from build123d import *

# Parameters (mm, degrees)
ESBO_O2_R                  = 1.65
RESSALTO_EXTRUS_O1_DEPTH   = 18
CORTE_EXTRUS_O1_DEPTH      = 47.043457733
CORTE_EXTRUS_O1_DEPTH_BACK = 47.043457733
ESBO_O3_R                  = 1.65
ESBO_O3_W                  = 19
ESBO_O3_H                  = 14
ESBO_O4_R                  = 1.6
CORTE_EXTRUS_O2_DEPTH      = 18


with BuildPart() as part:
    # Esboço2 → Ressalto-extrusão1 (new body)
    with BuildSketch(Plane.XY):
        with BuildLine():
            Line((0, 7), (-40, 7))
            Line((-40, 7), (-40, -7))
            Line((-40, -7), (-10.25, -7))
            Line((-10.25, -7), (-10.25, 0.7))
            Line((-10.25, 0.7), (-3.938273734, 0.7))
            ThreePointArc((-3.938273734, 0.7), (4, 0), (-3.938273734, -0.7))
            Line((-3.938273734, -0.7), (-9.75, -0.7))
            Line((-9.75, -0.7), (-9.75, -7))
            Line((-9.75, -7), (0, -7))
            ThreePointArc((0, -7), (7, 0), (0, 7))
        make_face()
        with Locations((-31, 0)):
            Circle(ESBO_O2_R, mode=Mode.SUBTRACT)
    extrude(amount=RESSALTO_EXTRUS_O1_DEPTH)

    # Esboço3 → Corte-extrusão1 (cut, two sides: drawn at the far end of the back side and taken through both)
    with BuildSketch(Plane.XZ.offset(7).offset(-CORTE_EXTRUS_O1_DEPTH_BACK)):
        with Locations((-6.844136867, 15)):
            Circle(ESBO_O3_R)
        with Locations((-30.5, 7)):
            Rectangle(ESBO_O3_W, ESBO_O3_H)
        with BuildLine():
            Line((7, 12), (-11, 12))
            ThreePointArc((-11, 12), (-15.242640687, 10.242640687), (-17, 6))
            Line((-17, 6), (-17, 0))
            Line((-17, 0), (7, 0))
            Line((7, 0), (7, 12))
        make_face()
    extrude(amount=CORTE_EXTRUS_O1_DEPTH + CORTE_EXTRUS_O1_DEPTH_BACK, mode=Mode.SUBTRACT)

    # Esboço4 → Corte-extrusão2 (cut)
    with BuildSketch(Plane.ZY.offset(21)):
        with Locations((4, 0)):
            Circle(ESBO_O4_R)
    extrude(amount=-CORTE_EXTRUS_O2_DEPTH, mode=Mode.SUBTRACT)


solid = part.part
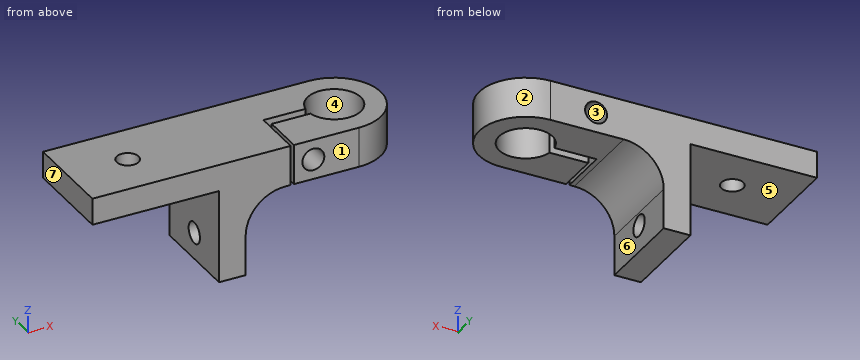
Here's how the part is built. I have some questions about the finished solid (model axes, mm). Face numbers are marked on the shaded views. A direction names the side the tool comes from. Coordinates: 2 decimals unless noted, no trailing zeros. Loops run counter-clockwise (first coordinate to the right, second up) from the corner with the lowest first, then second, coordinate; pieces in that order, holes last. Notation, with made-up numbers: (-19.75, -6) -> (9.25, -6) arc R18 ccw to (9.25, 16) -> close; hole circle Ø1 at (89.25, -35). An arc over 180 degrees is marked (long way). Use one line per item in the form item = value. Start each with the question number.
(1) We'd pull the mould along X, two halves only. Please class the marked faces 1, 2, 3 and 4: pulls with the +X half, pulls with the -X half, needs draft (parallel to the pull), parting line crosses it, or undercut.
(2) If we section it at B-B (y = 0): Please give me the cut outline in (x, z).
(3) If we section it at A-A (z = 15): Please give me the cut outline in (x, y).
(4) Please list where these lines run through material, in increasing order: line 1 along Y through (x, z) = (0, 15.65); line 2 along Z through (x, y) = (-22, -2.25); line 3 along Y through (x, z) = (-19.35, 4).
(5) If we section it at C-C (x = -31): Please give me the cut outline in (y, z), then the cut area to 3 significant figures.
(6) On a 3-axis mill with a long thin cutter (end or side, diameter ignored), from which of +Z, -Z, +X, -X, +Y, -Y can I reach the whole of each face in a straight line? I mean the marked faces 5, 6 and 7. Say none if no direction works.
(7) If we section it at D-D (y = -5.25): Please give me the cut outline in (x, z).
(8) Will these pins go through, and if not, where does the flat tip stop? pin 1 (1.5 mm diameter, centred on y = 2, z = 4.5, fed in from -X); pin 2 (3 mm diameter, centred on y = -5, z = 13.5, fed in from +X); pin 3 (6.5 mm diameter, centred on y = -3.5, z = 3.5, fed in from +X).
Verdict:
q1.face_1 = needs draft
q1.face_2 = pulls with the +X half
q1.face_3 = undercut
q1.face_4 = undercut
q2.outline = (-40, 14) -> (-32.65, 14) -> (-32.65, 18) -> (-40, 18) -> close; (-29.35, 14) -> (-21, 14) -> (-21, 5.6) -> (-17, 5.6) -> (-17, 6) arc R6 cw to (-11, 12) -> (-10.25, 12) -> (-10.25, 18) -> (-29.35, 18) -> close; (-21, 0) -> (-17, 0) -> (-17, 2.4) -> (-21, 2.4) -> close; (4, 12) -> (7, 12) -> (7, 18) -> (4, 18) -> close
q3.outline = (-40, -7) -> (-10.25, -7) -> (-10.25, 0.7) -> (-8.49, 0.7) -> (-8.49, 7) -> (-40, 7) -> close; (-9.75, -7) -> (-8.49, -7) -> (-8.49, -0.7) -> (-9.75, -0.7) -> close; (-5.19, -7) -> (0, -7) arc R7 ccw to (0, 7) -> (-5.19, 7) -> (-5.19, 0.7) -> (-3.94, 0.7) arc R4 cw (long way) to (-3.94, -0.7) -> (-5.19, -0.7) -> close; hole circle Ø3.3 at (-31, 0)
q4.line_1 = -7 to -4, 4 to 7
q4.line_2 = 14 to 18
q4.line_3 = -7 to -1.6, 1.6 to 7
q5.outline = (-7, 14) -> (-1.65, 14) -> (-1.65, 18) -> (-7, 18) -> close; (1.65, 14) -> (7, 14) -> (7, 18) -> (1.65, 18) -> close
q5.area = 42.8 mm²
q6.face_5 = -Z, -X, +Y, -Y
q6.face_6 = -Z, +X, +Y, -Y
q6.face_7 = +Z, -Z, -X, +Y, -Y
q7.outline = (-40, 14) -> (-21, 14) -> (-21, 0) -> (-17, 0) -> (-17, 6) arc R6 cw to (-11, 12) -> (-10.25, 12) -> (-10.25, 18) -> (-40, 18) -> close; (-9.75, 12) -> (4.63, 12) -> (4.63, 18) -> (-9.75, 18) -> close; hole circle Ø3.3 at (-6.84, 15)
q8.pin_1 = -21
q8.pin_2 = 6.06
q8.pin_3 = -16.95
